Autodesk Inventor part; units mm, degrees
ref_plane "XZ Plane" through (0, 0, 0) normal (0, 1, 0) x (-1, 0, 0)
ref_plane "XY Plane" through (0, 0, 0) normal (0, 0, 1) x (1, 0, 0)
sketch "Sketch1" plane through (0, 0, 0) normal (0, 0, 1) x (1, 0, 0)
  circle A0 centre (0, 0) radius 21.2725
  arc A1 (0, 33.9725) -> (-33.9725, 0) centre (0, 0) ccw
  line L0 (0, -33.9725) -> (-33.9725, -33.9725)
  line L1 (-33.9725, 0) -> (-33.9725, -33.9725)
  line L2 (0, 33.9725) -> (33.9725, 33.9725)
  line L3 (0, -33.9725) -> (33.9725, -33.9725)
  line L4 (33.9725, 0) -> (33.9725, -33.9725)
  line L5 (33.9725, 0) -> (33.9725, 33.9725)
  dimension "d0" = 42.545
  dimension "d1" = 67.945
extrude "Extrusion1" add sketch "Sketch1" along normal mid plane 12.7
sketch "Sketch2" plane through (-33.9725, -33.9725, 6.35) normal (-1, 0, 0) x (0, 0, 1)
  line L0 (0, 0) -> (-12.7, 0) construction
  line L1 (-6.35, 0) -> (-6.35, 33.9725) construction
  point P0 (-6.35, 10.16)
  dimension "d4" = 10.16
hole "Hole1" at (-33.9725, -23.8125, 0) direction (1, 0, 0) diameter 4.9784 depth 31.75 tip angle 118
ref_plane "Work Plane1" through (-9.525, 0, 0) normal (1, 0, 0) x (0, 1, 0)
sketch "Sketch3" plane through (33.9725, -33.9725, 6.35) normal (1, 0, 0) x (0, 0, -1)
  line L0 (0, 67.945) -> (12.7, 67.945) construction
  line L1 (6.35, 67.945) -> (6.35, 0) construction
  line L2 (0, 0) -> (12.7, 0) construction
  point P0 (6.35, 33.9725)
  point P1 (6.35, 61.595)
  point P2 (6.35, 6.35)
  dimension "d13" = 6.35
  dimension "d14" = 6.35
equation "\"d0\" = pipeDiameter"
equation "\"d1\" = pipeDiameter + 2 * outerRadius"
equation "\"pipeDiameter\" = 42.545"
equation "\"outerRadius\" = 12.7"
properties part number "gripperBracket"
Could you check a few things on this model? Use its own coordinates, in mm. A direction names the side the tool comes from. Give positions to 0.01 mm unless a question says otherwise; leave off trailing zeros. Loops run counter-clockwise (first coordinate to the right, second up) from the corner with the lowest first, then second, coordinate; pieces in that order, holes last. Notation, with made-up numbers: (-2, 52) -> (40, 52) arc R21 ccw to (40, 65) -> close; hole circle Ø1 at (-16.75, -39.5). An arc over 180 degrees is marked (long way). Answer as CSV lines item,"result". Start each with the question number.
(1) If we section it at C-C on y = -1: Write out the boundary of the cut face in (x, z).
(2) If we section it at B-B on z = 3.5: Write out the boundary of the cut face in (x, y) (1 decimal).
(3) I'm going to push flat-ended pins straight in: pin 1 Ø1.5 at (y, z) = (7.5, -0.5) entering from -X; pin 2 Ø4.5 at (y, z) = (-23.81, 0) entering from -X; pin 3 Ø1.5 at (y, z) = (16, -1) entering from -X. Where does each tip first touch, or does it pass through?
(4) We'd pull the mould along X, two halves only. Please class faces 1 (the flat face through (0, -33.972, 0)), 2 (the cylindrical face through (-16.881, 12.944, -0.089)), 3 (the flat face through (33.972, 0, 0)): released by +X, released by -X, zero draft, split by the parting line, or undercut.
(5) If we section it at A-A on x = -3.5: Write out the boundary of the cut face in (y, z).
(6) I need wall thicknesses on probe 1 along Y at (x, z) = (0, 2.25); probe 2 along Y at (x, z) = (-10, 0); probe 3 along X at (y, z) = (21.5, -2.75). Which ranges of each line are inside material? Lowest first, please.
(7) Which directions (+Z, -Z, +X, -X, +Y, -Y) give clear straight access to the entire face, cutting with the end or side of a thin tool? Please do faces 4 (the flat face through (22, 0, 6.35)), 5 (the cylindrical face through (-17.875, -21.382, -0.54)).
(8) If we section it at D-D on x = 11.5: Write out the boundary of the cut face in (y, z).
Computed:
1,outline,"(-33.97, -6.35) -> (-21.25, -6.35) -> (-21.25, 6.35) -> (-33.97, 6.35) -> close; (21.25, -6.35) -> (33.97, -6.35) -> (33.97, 6.35) -> (21.25, 6.35) -> close"
2,outline,"(-34, -34) -> (34, -34) -> (34, 34) -> (0, 34) arc R34 ccw to (-34, 0) -> close; hole circle Ø42.5 at (0, 0)"
3,pin 1,"stops at x = -33.3"
3,pin 2,"stops at x = -2.08"
3,pin 3,"stops at x = -30.36"
4,face 1,"zero draft"
4,face 2,"undercut"
4,face 3,"released by +X"
5,outline,"(-33.97, -6.35) -> (-20.98, -6.35) -> (-20.98, 6.35) -> (-33.97, 6.35) -> close; (20.98, -6.35) -> (33.79, -6.35) -> (33.79, 6.35) -> (20.98, 6.35) -> close; hole circle Ø4.98 at (-23.81, 0)"
6,probe 1,"y = -33.97 to -21.27, 21.27 to 33.97"
6,probe 2,"y = -33.97 to -26.3, -21.32 to -18.78, 18.78 to 32.47"
6,probe 3,"x = -26.3 to 33.97"
7,face 4,"+Z, +X, -X, +Y, -Y"
7,face 5,"-X"
8,outline,"(-33.97, -6.35) -> (-17.9, -6.35) -> (-17.9, 6.35) -> (-33.97, 6.35) -> close; (17.9, -6.35) -> (33.97, -6.35) -> (33.97, 6.35) -> (17.9, 6.35) -> close"
